from build123d import *

# Parameters (mm, degrees)
SKETCH1_R           = 1.65
BOSS_EXTRUDE1_DEPTH = 8
SKETCH2_W           = 10.32
SKETCH2_H           = 9
CUT_EXTRUDE1_DEPTH  = 2.4
SKETCH3_W           = 10.32
SKETCH3_H           = 9
CUT_EXTRUDE2_DEPTH  = 2.4
BOSS_EXTRUDE2_DEPTH = 8
SKETCH7_W           = 76.8
SKETCH7_H           = 1
CUT_EXTRUDE3_DEPTH  = 68.43727806
SKETCH9_W           = 10.32
SKETCH9_H           = 0.1
CUT_EXTRUDE4_DEPTH  = 10
SKETCH10_R          = 1.6
SKETCH10_W          = 1.25
SKETCH10_H          = 66.8
SKETCH10_W_2        = 0.75
SKETCH10_H_2        = 76.8
CUT_EXTRUDE5_DEPTH  = 6


with BuildPart() as part:
    # Sketch1 → Boss-Extrude1 (new body)
    with BuildSketch(Plane(origin=(0, 0, 0), x_dir=(1, 0, 0), z_dir=(0, 1, 0))):
        Polygon((-37.890672074, -44.431484199), (-30.550672074, -44.431484199), (-30.550672074, -45.431484199), (-20.230672074, -45.431484199), (-20.230672074, -44.431484199), (-12.890672074, -44.431484199), (-12.890672074, 4.468515801), (-7.890672074, 4.468515801), (-7.890672074, -54.431484199), (-42.890672074, -54.431484199), (-42.890672074, 4.468515801), (-37.890672074, 4.468515801), align=None)
        with Locations(Location((-25.390672074, -50.431484199, 0), (0, 0, 270))):
            Circle(SKETCH1_R, mode=Mode.SUBTRACT)
    extrude(amount=BOSS_EXTRUDE1_DEPTH)

    # Sketch2 → Cut-Extrude1 (cut)
    with BuildSketch(Plane(origin=(0, 8, 0), x_dir=(1, 0, 0), z_dir=(0, 1, 0))):
        with Locations((-25.390672074, -49.931484199)):
            Rectangle(SKETCH2_W, SKETCH2_H)
    extrude(amount=-CUT_EXTRUDE1_DEPTH, mode=Mode.SUBTRACT)

    # Sketch3 → Cut-Extrude2 (cut)
    with BuildSketch(Plane.XZ):
        with Locations((-25.390672074, 49.931484199)):
            Rectangle(SKETCH3_W, SKETCH3_H)
    extrude(amount=-CUT_EXTRUDE2_DEPTH, mode=Mode.SUBTRACT)

    # Sketch6 → Boss-Extrude2 (add)
    with BuildSketch(Plane.XZ):
        Polygon((-37.890672074, -22.368515801), (-37.890672074, -4.468515801), (-42.890672074, -4.468515801), (-42.890672074, 54.431484199), (-44.890672074, 54.431484199), (-44.890672074, -10.768515801), (-44.890672074, -22.368515801), align=None)
        Polygon((-7.890672074, -4.468515801), (-12.890672074, -4.468515801), (-12.890672074, -22.368515801), (-5.890672074, -22.368515801), (-5.890672074, -10.768515801), (-5.890672074, 54.431484199), (-7.890672074, 54.431484199), align=None)
    extrude(amount=-BOSS_EXTRUDE2_DEPTH)

    # Sketch7 → Cut-Extrude3 (cut, through all)
    with BuildSketch(Plane(origin=(-5.890672074, 0, 0), x_dir=(0, 0, -1), z_dir=(1, 0, 0))):
        with Locations((-16.031484199, 7.5)):
            Rectangle(SKETCH7_W, SKETCH7_H)
        with Locations((-16.031484199, 0.5)):
            Rectangle(SKETCH7_W, SKETCH7_H)
    extrude(amount=-CUT_EXTRUDE3_DEPTH, mode=Mode.SUBTRACT)

    # Sketch9 → Cut-Extrude4 (cut)
    with BuildSketch(Plane.XY.offset(54.431484199)):
        with Locations((-25.390672074, 5.55)):
            Rectangle(SKETCH9_W, SKETCH9_H)
        with Locations((-25.390672074, 2.45)):
            Rectangle(SKETCH9_W, SKETCH9_H)
    extrude(amount=-CUT_EXTRUDE4_DEPTH, mode=Mode.SUBTRACT)

    # Sketch10 → Cut-Extrude5 (cut)
    with BuildSketch(Plane(origin=(0, 7, 0), x_dir=(1, 0, 0), z_dir=(0, 1, 0))):
        with Locations(Location((-41.640672074, 19.168515801, 0), (0, 0, 270))):
            Circle(SKETCH10_R)
        with Locations(Location((-9.140672074, 19.168515801, 0), (0, 0, 270))):
            Circle(SKETCH10_R)
        with Locations((-38.515672074, -11.031484199)):
            Rectangle(SKETCH10_W, SKETCH10_H)
        with Locations((-12.265672074, -11.031484199)):
            Rectangle(SKETCH10_W, SKETCH10_H)
        with Locations((-6.265672074, -16.031484199)):
            Rectangle(SKETCH10_W_2, SKETCH10_H_2)
        with Locations((-44.515672074, -16.031484199)):
            Rectangle(SKETCH10_W_2, SKETCH10_H_2)
    extrude(amount=-CUT_EXTRUDE5_DEPTH, mode=Mode.SUBTRACT)


solid = part.part
Can you work these out from the model? Positions are in its coordinate system, mm. A direction names the side the tool comes from. Coordinates: 2 decimals unless noted, no trailing zeros. Order: outer loops, then holes, each group sorted by start corner. A loop starts at its lowest first (then second) coordinate and runs counter-clockwise, first axis right, second up. Notation, with made-up numbers: M -29,62.5 L -20,62.5 A18 cw -20,72.5 Z; hole C -1.75,-13.5 d2. An arc over 180 degrees is marked long. Write item = value, one per line.
(1) If we mould it in two halves opening along X, with no side actions, what happens to faces 1 (the face through (-25, 4, 54.431)), 2 (the face through (-26.39, 3.98, 49.12)), 3 (the face through (-44.141, 4, 17)), 4 (the face through (-24, 5.5, 49))? For each: pulls with the +X half, pulls with the -X half, needs draft (parallel to the pull), parting line crosses it, or undercut.
Results are:
face_1 = needs draft
face_2 = undercut
face_3 = pulls with the -X half
face_4 = undercut
(2) For faces 5 (the face through (-10, 1, 25)), 6 (the face through (-24, 2.5, 49)), 7 (the face through (-30.551, 2, 49)), 8 (the face through (-35, 4, 44.431)), which set-ups out of +Z, -Z, +X, -X, +Y, -Y let a thin tool reach every point of the face, with its end or its side?
Results are:
face_5 = +Z, -Z, +X, -X, -Y
face_6 = +Z, -Z, -Y
face_7 = -Z
face_8 = -Z, +Y, -Y
(3) I need wall thicknesses on line 1 along X through (y, z) = (4.4, 2.5); line 2 along X through (y, z) = (2.35, 49); line 3 along Z through (x, y) = (-39, 3.45). Which ranges of each line are inside material? Lowest first, please. Write a range as [from, to].
Results are:
line_1 = [-44.14, -39.14], [-11.64, -6.64]
line_2 = [-44.14, -30.55], [-20.23, -6.64]
line_3 = [44.43, 54.43]
(4) Suppose I cut it at A-A on z = -11.5. Please give me the cut outline in (x, y).
Results are:
outline = M -44.14,1 L -39.14,1 L -39.14,7 L -44.14,7 Z; M -11.64,1 L -6.64,1 L -6.64,7 L -11.64,7 Z
(5) Suppose I cut it at C-C on x = -36. Please give me the cut outline in (y, z).
Results are:
outline = M 1,44.43 L 7,44.43 L 7,54.43 L 1,54.43 Z
(6) Suppose I cut it at D-D on x = -22.5. Please give me the cut outline in (y, z), plus the area to 3 significant figures.
Results are:
outline = M 2.5,45.43 L 5.5,45.43 L 5.5,54.43 L 2.5,54.43 Z
area = 27.0 mm2
(7) Suppose I cut it at B-B on y = 4.4. Please give me the cut outline in (x, z).
Results are:
outline = M -44.14,-22.37 L -39.14,-22.37 L -39.14,44.43 L -30.55,44.43 L -30.55,45.43 L -20.23,45.43 L -20.23,44.43 L -11.64,44.43 L -11.64,-22.37 L -6.64,-22.37 L -6.64,54.43 L -44.14,54.43 Z; hole C -41.64,-19.17 d3.2; hole C -25.39,50.43 d3.3; hole C -9.14,-19.17 d3.2
(8) For pin 1 Ø2.5 at (x, z) = (-26, 48.5) entering from +Y; pin 2 Ø1.5 at (x, y) = (-34, 6.5) entering from -Z; pin 3 Ø3 at (x, z) = (-41.64, -19.17) entering from +Y; pin 4 Ø2.5 at (x, y) = (-28, 4) entering from -Z, each with a flat end and sliding along its axis, tell me the tip position at first contact or that it passes through.
Results are:
pin_1 = 5.5
pin_2 = 44.43
pin_3 = through
pin_4 = 45.43
